Read the model definition and answer for the solid it produces. Units are mm, in the model's axes. A direction names the side the tool comes from. Give positions to 0.01 mm unless a question says otherwise; leave off trailing zeros. Write item = value, one per line. Start each with the question number.
from build123d import *

# Parameters (mm, degrees)
SKETCH1_R                                       = 32.75
SKETCH1_R_2                                     = 15.25
SKETCH1_R_3                                     = 4.25
BOSS_EXTRUDE1_DEPTH                             = 12
SKETCH1_4_R                                     = 4.25
CUT_EXTRUDE2_DEPTH                              = 95.16807527
CUT_EXTRUDE3_START                              = 6
SKETCH1_6_R                                     = 32.75
SKETCH1_6_R_2                                   = 4.25
SKETCH1_6_R_3                                   = 15.25
CUT_EXTRUDE3_DEPTH                              = 89.16807527
CHAMFER1_SIZE                                   = 1
CHAMFER2_SIZE                                   = 0.5
CSK_FOR_M8_FLAT_HEAD_MACHINE_SCREW1_D           = 9
CSK_FOR_M8_FLAT_HEAD_MACHINE_SCREW1_CSINK_D     = 18
CSK_FOR_M8_FLAT_HEAD_MACHINE_SCREW1_CSINK_ANGLE = 90


with BuildPart() as part:
    # Sketch1 → Boss-Extrude1 (new body)
    # profile 1 of 9: a face of its own
    with BuildSketch(Plane(origin=(0, 0, 0), x_dir=(1, 0, 0), z_dir=(0, 1, 0))):
        with BuildLine():
            Line((-40, -80.42), (40, -80.42))
            ThreePointArc((40, -80.42), (45.303300859, -78.223300859), (47.5, -72.92))
            Line((47.5, -72.92), (47.5, 32.08))
            ThreePointArc((47.5, 32.08), (45.303300859, 37.383300859), (40, 39.58))
            Line((40, 39.58), (-40, 39.58))
            ThreePointArc((-40, 39.58), (-45.303300859, 37.383300859), (-47.5, 32.08))
            Line((-47.5, 32.08), (-47.5, -72.92))
            ThreePointArc((-47.5, -72.92), (-45.303300859, -78.223300859), (-40, -80.42))
        make_face()
        Circle(SKETCH1_R, mode=Mode.SUBTRACT)
        with Locations((0, -58.34)):
            Circle(SKETCH1_R_2, mode=Mode.SUBTRACT)
        with BuildLine():
            ThreePointArc((46, 32.08), (40, 38.08), (34, 32.08))
            Line((34, 32.08), (34, -72.92))
            ThreePointArc((34, -72.92), (40, -78.92), (46, -72.92))
            Line((46, -72.92), (46, 32.08))
        make_face(mode=Mode.SUBTRACT)
        with BuildLine():
            ThreePointArc((-34, 32.08), (-40, 38.08), (-46, 32.08))
            Line((-46, 32.08), (-46, -72.92))
            ThreePointArc((-46, -72.92), (-40, -78.92), (-34, -72.92))
            Line((-34, -72.92), (-34, 32.08))
        make_face(mode=Mode.SUBTRACT)
    # profile 2 of 9: a face of its own
    with BuildSketch(Plane(origin=(0, 0, 0), x_dir=(1, 0, 0), z_dir=(0, 1, 0))):
        Circle(SKETCH1_R)
        Circle(SKETCH1_R_3, mode=Mode.SUBTRACT)
    # profile 3 of 9: a face of its own
    with BuildSketch(Plane(origin=(0, 0, 0), x_dir=(1, 0, 0), z_dir=(0, 1, 0))):
        with Locations((0, -58.34)):
            Circle(SKETCH1_R_2)
        with Locations((0, -58.34)):
            Circle(SKETCH1_R_3, mode=Mode.SUBTRACT)
    # profile 4 of 9: a face of its own
    with BuildSketch(Plane(origin=(0, 0, 0), x_dir=(1, 0, 0), z_dir=(0, 1, 0))):
        with BuildLine():
            Line((-34, -72.92), (-34, 32.08))
            ThreePointArc((-34, 32.08), (-40, 38.08), (-46, 32.08))
            Line((-46, 32.08), (-46, -72.92))
            ThreePointArc((-46, -72.92), (-40, -78.92), (-34, -72.92))
        make_face()
        with BuildLine():
            ThreePointArc((-43.25, -72.92), (-40, -76.17), (-36.75, -72.92))
            Line((-36.75, -72.92), (-36.75, 32.08))
            ThreePointArc((-36.75, 32.08), (-40, 35.33), (-43.25, 32.08))
            Line((-43.25, 32.08), (-43.25, -72.92))
        make_face(mode=Mode.SUBTRACT)
    # profile 5 of 9: a face of its own
    with BuildSketch(Plane(origin=(0, 0, 0), x_dir=(1, 0, 0), z_dir=(0, 1, 0))):
        with BuildLine():
            Line((46, -72.92), (46, 32.08))
            ThreePointArc((46, 32.08), (40, 38.08), (34, 32.08))
            Line((34, 32.08), (34, -72.92))
            ThreePointArc((34, -72.92), (40, -78.92), (46, -72.92))
        make_face()
        with BuildLine():
            ThreePointArc((36.75, -72.92), (40, -76.17), (43.25, -72.92))
            Line((43.25, -72.92), (43.25, 32.08))
            ThreePointArc((43.25, 32.08), (40, 35.33), (36.75, 32.08))
            Line((36.75, 32.08), (36.75, -72.92))
        make_face(mode=Mode.SUBTRACT)
    # profile 6 of 9: a face of its own
    with BuildSketch(Plane(origin=(0, 0, 0), x_dir=(1, 0, 0), z_dir=(0, 1, 0))):
        with BuildLine():
            Line((36.75, 32.08), (36.75, -72.92))
            ThreePointArc((36.75, -72.92), (40, -76.17), (43.25, -72.92))
            Line((43.25, -72.92), (43.25, 32.08))
            ThreePointArc((43.25, 32.08), (40, 35.33), (36.75, 32.08))
        make_face()
    # profile 7 of 9: a face of its own
    with BuildSketch(Plane(origin=(0, 0, 0), x_dir=(1, 0, 0), z_dir=(0, 1, 0))):
        with BuildLine():
            Line((-43.25, 32.08), (-43.25, -72.92))
            ThreePointArc((-43.25, -72.92), (-40, -76.17), (-36.75, -72.92))
            Line((-36.75, -72.92), (-36.75, 32.08))
            ThreePointArc((-36.75, 32.08), (-40, 35.33), (-43.25, 32.08))
        make_face()
    # profile 8 of 9: a face of its own
    with BuildSketch(Plane(origin=(0, 0, 0), x_dir=(1, 0, 0), z_dir=(0, 1, 0))):
        Circle(SKETCH1_R_3)
    # profile 9 of 9: a face of its own
    with BuildSketch(Plane(origin=(0, 0, 0), x_dir=(1, 0, 0), z_dir=(0, 1, 0))):
        with Locations((0, -58.34)):
            Circle(SKETCH1_R_3)
    extrude(amount=BOSS_EXTRUDE1_DEPTH)

    # Sketch1_4 → Cut-Extrude2 (cut, through all)
    with BuildSketch(Plane(origin=(0, 0, 0), x_dir=(1, 0, 0), z_dir=(0, 1, 0))):
        with BuildLine():
            Line((36.75, 32.08), (36.75, -72.92))
            ThreePointArc((36.75, -72.92), (40, -76.17), (43.25, -72.92))
            Line((43.25, -72.92), (43.25, 32.08))
            ThreePointArc((43.25, 32.08), (40, 35.33), (36.75, 32.08))
        make_face()
        with Locations(Location((0, 0, 0), (0, 0, 270))):
            Circle(SKETCH1_4_R)
        with Locations(Location((0, -58.34, 0), (0, 0, 270))):
            Circle(SKETCH1_4_R)
        with BuildLine():
            Line((-43.25, 32.08), (-43.25, -72.92))
            ThreePointArc((-43.25, -72.92), (-40, -76.17), (-36.75, -72.92))
            Line((-36.75, -72.92), (-36.75, 32.08))
            ThreePointArc((-36.75, 32.08), (-40, 35.33), (-43.25, 32.08))
        make_face()
    extrude(amount=CUT_EXTRUDE2_DEPTH, mode=Mode.SUBTRACT)

    # Sketch1_6 → Cut-Extrude3 (cut, through all)
    # profile 1 of 2: a face of its own
    with BuildSketch(Plane(origin=(0, 0, 0), x_dir=(1, 0, 0), z_dir=(0, 1, 0)).offset(CUT_EXTRUDE3_START)):
        with Locations(Location((0, 0, 0), (0, 0, 270))):
            Circle(SKETCH1_6_R)
        with Locations(Location((0, 0, 0), (0, 0, 270))):
            Circle(SKETCH1_6_R_2, mode=Mode.SUBTRACT)
    # profile 2 of 2: a face of its own
    with BuildSketch(Plane(origin=(0, 0, 0), x_dir=(1, 0, 0), z_dir=(0, 1, 0)).offset(CUT_EXTRUDE3_START)):
        with Locations(Location((0, -58.34, 0), (0, 0, 270))):
            Circle(SKETCH1_6_R_3)
        with Locations(Location((0, -58.34, 0), (0, 0, 270))):
            Circle(SKETCH1_6_R_2, mode=Mode.SUBTRACT)
    extrude(amount=CUT_EXTRUDE3_DEPTH, mode=Mode.SUBTRACT)

    # Chamfer1
    chamfer1_edges = [part.edges().sort_by_distance(p)[0] for p in [
        (0, 12, -32.75),
        (0, 12, 43.09),
    ]]
    chamfer(chamfer1_edges, length=CHAMFER1_SIZE)

    # Chamfer2
    chamfer2_edges = [part.edges().sort_by_distance(p)[0] for p in [
        (-45.303300859, 0, 78.223300859),
        (45.303300859, 12, 78.223300859),
        (-47.5, 0, 20.42),
        (-45.303300859, 0, -37.383300859),
        (0, 0, -39.58),
        (45.303300859, 0, -37.383300859),
        (47.5, 0, 20.42),
        (45.303300859, 0, 78.223300859),
        (0, 0, 80.42),
        (47.5, 12, 20.42),
        (45.303300859, 12, -37.383300859),
        (0, 12, -39.58),
        (-45.303300859, 12, -37.383300859),
        (36.75, 0, 20.42),
        (40, 0, 76.17),
        (43.25, 12, 20.42),
        (40, 0, -35.33),
        (-47.5, 12, 20.42),
        (36.75, 12, 20.42),
        (40, 12, 76.17),
        (40, 12, -35.33),
        (43.25, 0, 20.42),
        (0, 0, -4.25),
        (-45.303300859, 12, 78.223300859),
        (0, 0, 54.09),
        (-43.25, 0, 20.42),
        (-40, 0, 76.17),
        (0, 12, 80.42),
        (-36.75, 12, 20.42),
        (-40, 0, -35.33),
        (-43.25, 12, 20.42),
        (-40, 12, 76.17),
        (-40, 12, -35.33),
        (-36.75, 0, 20.42),
        (0, 6, -4.25),
        (0, 6, 54.09),
    ]]
    chamfer(chamfer2_edges, length=CHAMFER2_SIZE)

    # CSK for M8 Flat Head Machine Screw1 (through all)
    with Locations(Plane(origin=(0, 0, 0), x_dir=(-1, 0, 0), z_dir=(0, -1, 0))):
        with Locations((0, 0), (0, -58.34)):
            CounterSinkHole(CSK_FOR_M8_FLAT_HEAD_MACHINE_SCREW1_D / 2, CSK_FOR_M8_FLAT_HEAD_MACHINE_SCREW1_CSINK_D / 2, counter_sink_angle=CSK_FOR_M8_FLAT_HEAD_MACHINE_SCREW1_CSINK_ANGLE)


solid = part.part
1) Find section A-A on x = 0. Count the separate pieces of the cut face and the enclosed holes in it, plus the area to 3 significant figures.
2) For faces 4 (the face through (-43.25, 6, 20)), 5 (the face through (-39.93, 0.36, -35.47)), 6 (the face through (40.074, 11.635, 76.305)), determine the directions among +Z, -Z, +X, -X, +Y, -Y from which every point of the face is accessible in a straight line to the end or side of a thin tool.
3) For a pull along Z with two mould halves and no side action, classify faces 1 (the face through (44.99, 0.135, 78.021)), 2 (the face through (1, 6, -39.58)), 3 (the face through (2.177, 4.282, 62.526)) as pulls with the +Z half, pulls with the -Z half, needs draft (parallel to the pull), parting line crosses it, or undercut.
4) Each of these flat-tipped pins is pushed along its axis until it touches: P1, Ø15, axis at x = -2, z = 58.5, coming from the +Y side; P2, Ø5.5, axis at x = 0, z = 58.34, coming from the +Y side. Where does it stop, or does it pass through?
5) Find the intervals of material crossed by probe 1 along X at (y, z) = (2.25, 50); probe 2 along Z at (x, y) = (0, 5.5); probe 3 along Z at (x, y) = (0, 9.25), in increasing order. Write a range as [from, to].
Numbers:
q1.separate_pieces = 3
q1.enclosed_holes = 0
q1.area = 713 mm2
q2.face_4 = +Y, -Y
q2.face_5 = -Y
q2.face_6 = +Y
q3.face_1 = pulls with the +Z half
q3.face_2 = pulls with the -Z half
q3.face_3 = undercut
q4.P1 = 6
q4.P2 = through
q5.probe_1 = [-47.5, -43.25], [-36.75, 36.75], [43.25, 47.5]
q5.probe_2 = [-39.58, -4.5], [4.5, 53.84], [62.84, 80.42]
q5.probe_3 = [-39.58, -32.75], [32.75, 43.09], [73.59, 80.42]
